from build123d import *

# Parameters (mm, degrees)
BOSS_EXTRUDE1_DEPTH = 1.5
SKETCH2_R           = 4
CUT_EXTRUDE2_DEPTH  = 2.5
CHAMFER1_SIZE       = 1
FILLET1_R           = 0.3


with BuildPart() as part:
    # Sketch1 → Boss-Extrude1 (new body)
    with BuildSketch(Plane(origin=(0, 0, 0), x_dir=(1, 0, 0), z_dir=(0, 1, 0))):
        with BuildLine():
            Line((-7, 6), (7, 6))
            ThreePointArc((7, 6), (13, 0), (7, -6))
            Line((7, -6), (-7, -6))
            ThreePointArc((-7, -6), (-13, 0), (-7, 6))
        make_face()
    extrude(amount=BOSS_EXTRUDE1_DEPTH)

    # Sketch2 → Cut-Extrude2 (cut, through all)
    with BuildSketch(Plane(origin=(0, 0, 0), x_dir=(1, 0, 0), z_dir=(0, 1, 0))):
        with Locations(Location((-7, 0, 0), (0, 0, 270))):  # turned: the seam where the file's is
            Circle(SKETCH2_R)
        with Locations(Location((7, 0, 0), (0, 0, 270))):  # turned: the seam where the file's is
            Circle(SKETCH2_R)
    extrude(amount=CUT_EXTRUDE2_DEPTH, mode=Mode.SUBTRACT)

    # Chamfer1
    chamfer1_edges = [part.edges().sort_by_distance(p)[0] for p in [
        (-7, 1.5, -4),
        (7, 1.5, -4),
    ]]
    chamfer(chamfer1_edges, length=CHAMFER1_SIZE)

    # Fillet1
    fillet1_edges = [part.edges().sort_by_distance(p)[0] for p in [
        (13, 1.5, 0),
        (0, 1.5, -6),
        (-7, 0.5, -4),
        (7, 1.5, -5),
        (-7, 1.5, -5),
        (7, 0.5, -4),
        (-13, 1.5, 0),
        (0, 0, -6),
        (13, 0, 0),
        (0, 0, 6),
        (-13, 0, 0),
        (0, 1.5, 6),
    ]]
    fillet(fillet1_edges, radius=FILLET1_R)


solid = part.part
CAD build for the part. Positions are in the model's coordinates, mm. Give positions to 0.01 mm unless a question says otherwise; leave off trailing zeros. Loops run counter-clockwise (first coordinate to the right, second up) from the corner with the lowest first, then second, coordinate; pieces in that order, holes last. Notation, with made-up numbers: M -5.75,35.5 L 49.25,35.5 A24 cw 49.25,65.5 Z; hole C 41,50.5 d2. An arc over 180 degrees is marked long. One line per question, with ' | ' between items. Start each with the question number.
1. Probe L1, parallel to X at y = 0.15, z = 0; L2, parallel to X at y = 0.6, z = -1; L3, parallel to Z at x = -7, y = 0.25. List the from-to ranges inside material, lowest first. Write a range as from..to.
2. Two-plate mould, pull along X, no slides. Class faces 1 (the face through (7.176, 0.185, -3.996)), 2 (the face through (-13, 1, 0)), 3 (the face through (13, 1, 0)): pulls with the +X half, pulls with the -X half, needs draft (parallel to the pull), parting line crosses it, or undercut.
3. Flat gauge pin, fed straight in: pin 1 (7 mm diameter, centred on x = -7, z = 0, fed in from -Y). Where does the tip first touch, or does it go through?
4. Saw through at A-A on y = 0.9. Give the cut face in (x, z), plus the area to 3 significant figures.
5. Saw through at B-B on z = 0. State how many separate pieces and enclosed holes the cut face has, plus the area to 3 significant figures.
Result sheet:
1) L1: x = -12.96..-11, -3..3, 11..12.96 | L2: x = -12.92..-10.98, -3.02..3.02, 10.98..12.92 | L3: z = -6..-4, 4..6
2) face 1: undercut | face 2: pulls with the -X half | face 3: pulls with the +X half
3) pin 1: passes through
4) outline: M -7,-6 L 7,-6 A6 ccw 7,6 L -7,6 A6 ccw Z; hole C -7,0 d8.8; hole C 7,0 d8.8 | area: 159 mm^2
5) separate pieces: 3 | enclosed holes: 0 | area: 12.9 mm^2
